Autodesk Fusion 360 part; units mm, degrees
sketch "Esquisse1" plane through (0, 0, 0) normal (0, 0, 1) x (1, 0, 0)
  line L0 (-30, 40) -> (30, 40)
  line L1 (30, 40) -> (30, -40)
  line L2 (30, -40) -> (-30, -40)
  line L3 (-30, -40) -> (-30, 40)
  line L4 (-30, 40) -> (30, -40) construction
  line L5 (30, 40) -> (-30, -40) construction
  dimension "d1" = 60
  dimension "d2" = 80
extrude "Extrusion1" add sketch "Esquisse1" along normal blind 5
sketch "Esquisse2" plane through (0, 0, 5) normal (0, 0, 1) x (-1, 0, 0)
  line L0 (30, 40) -> (-30, 40)
  line L1 (-30, 40) -> (-30, -40)
  line L2 (-30, -40) -> (30, -40)
  line L3 (30, -40) -> (30, 40)
  line L4 (4.5, -29.5) -> (-4.5, -29.5)
  line L5 (-4.5, -29.5) -> (-4.5, 29.5)
  line L6 (-4.5, 29.5) -> (4.5, 29.5)
  line L7 (4.5, 29.5) -> (4.5, -29.5)
  line L8 (4.5, -29.5) -> (-4.5, 29.5) construction
  line L9 (-4.5, -29.5) -> (4.5, 29.5) construction
  dimension "d5" = 59
  dimension "d6" = 9
extrude "Extrusion2" add sketch "Esquisse2" along normal blind 17 contours L4 L5 L6 L7
sketch "Esquisse3" plane through (0, 0, 22) normal (0, 0, 1) x (-1, 0, 0)
  line L0 (4.5, 29.5) -> (-4.5, 29.5)
  line L1 (-4.5, 29.5) -> (-4.5, -29.5)
  line L2 (-4.5, -29.5) -> (4.5, -29.5)
  line L3 (4.5, -29.5) -> (4.5, 29.5)
  line L4 (9.5, -29.5) -> (-9.5, -29.5)
  line L5 (-9.5, -29.5) -> (-9.5, 29.5)
  line L6 (-9.5, 29.5) -> (9.5, 29.5)
  line L7 (9.5, 29.5) -> (9.5, -29.5)
  line L8 (9.5, -29.5) -> (-9.5, 29.5) construction
  line L9 (-9.5, -29.5) -> (9.5, 29.5) construction
  dimension "d9" = 59
  dimension "d10" = 19
extrude "Extrusion3" add sketch "Esquisse3" along normal blind 3
sketch "Esquisse4" plane through (0, 0, 25) normal (0, 0, 1) x (-1, 0, 0)
  line L0 (9.5, 29.5) -> (-9.5, 29.5)
  line L1 (-9.5, 29.5) -> (-9.5, -29.5)
  line L2 (-9.5, -29.5) -> (9.5, -29.5)
  line L3 (9.5, -29.5) -> (9.5, 29.5)
  line L4 (-9.5, 29.5) -> (9.5, 29.5)
  line L5 (9.5, 29.5) -> (9.5, 19.5)
  line L6 (9.5, 19.5) -> (-9.5, 19.5)
  line L7 (-9.5, 19.5) -> (-9.5, 29.5)
  dimension "d13" = 10
extrude "Extrusion4" add sketch "Esquisse4" along normal blind 10 from surface at -7.5 contours L0 L1 L3 L4 L5 L6 L7
chamfer "Chanfrein5" distance 4 angle 45 1 edges at (4.5, 0, 5)
chamfer "Chanfrein6" distance 4 angle 45 1 edges at (-4.5, 0, 5)
sketch "Esquisse10" plane through (0, -29.5, 0) normal (0, -1, 0) x (1, 0, 0)
  line L0 (9.5, 17.5) -> (9.5, 27.5)
  line L1 (-9.5, 27.5) -> (-9.5, 17.5)
  line L2 (-4.5, 17.5) -> (-4.5, 9)
  line L3 (-4.5, 9) -> (-8.5, 5)
  line L4 (-8.5, 5) -> (8.5, 5)
  line L5 (8.5, 5) -> (4.5, 9)
  line L6 (4.5, 9) -> (4.5, 17.5)
  line L7 (0, 25) -> (0, 23)
  line L8 (0, 23) -> (-3.25, 23)
  line L9 (-3.25, 23) -> (3.25, 23)
  line L10 (3.25, 23) -> (3.25, 14.5)
  line L11 (3.25, 14.5) -> (-3.25, 14.5)
  line L12 (-3.25, 14.5) -> (-3.25, 23)
  line L13 (-3.25, 23) -> (3.25, 23)
  line L14 (3.25, 23) -> (3.25, 19.5)
  line L15 (3.25, 19.5) -> (-3.25, 19.5)
  line L16 (-3.25, 19.5) -> (-3.25, 23)
  line L17 (4.5, 17.5) -> (9.5, 17.5)
  line L18 (9.5, 27.5) -> (-9.5, 27.5)
  line L19 (-9.5, 27.5) -> (9.5, 27.5)
  line L20 (-9.5, 17.5) -> (-4.5, 17.5)
  point P0 (0, 25)
  point P1 (0, 23)
  dimension "d33" = 6.5
  dimension "d34" = 3.5
  dimension "d35" = 8.5
  dimension "d46" = 4.5
extrude "Extrusion9" add sketch "Esquisse10" along normal blind 6 contours L8 L9 L10 L12 L13 L14 L15 L16
extrude "Extrusion10" add sketch "Esquisse10" along normal blind 4 from surface at 5 contours L8 L9 L10 L12 L13 L14 L15 L16 | L10 L11 L12 L15
extrude "Extrusion11" add 2 faces at (7.8333, 13.1667, 22) (-7.8333, 13.1667, 22) along direction (0, 0, -1) blind 4
sketch "Esquisse11" plane through (0, 0, 5) normal (0, 0, 1) x (-1, 0, 0)
  line L0 (8.5, -29.5) -> (-8.5, -29.5)
  line L1 (-8.5, -29.5) -> (-8.5, 29.5)
  line L2 (-8.5, 29.5) -> (8.5, 29.5)
  line L3 (8.5, 29.5) -> (8.5, -29.5)
  line L4 (30, 40) -> (-30, 40)
  line L5 (-30, 40) -> (-30, -40)
  line L6 (-30, -40) -> (30, -40)
  line L7 (30, -40) -> (30, 40)
  circle A0 centre (19, -19) radius 1.55
  circle A1 centre (19, 18) radius 1.55
  circle A2 centre (-19, -19) radius 1.55
  circle A3 centre (-19, 18) radius 1.55
  dimension "d47" = 3.1
  dimension "d48" = 3.1
  dimension "d49" = 3.1
  dimension "d50" = 3.1
  dimension "d51" = 37
  dimension "d52" = 37
  dimension "d53" = 11
  dimension "d54" = 11
  dimension "d55" = 11
  dimension "d56" = 11
  dimension "d57" = 22
  dimension "d58" = 22
extrude "Extrusion12" cut sketch "Esquisse11" against normal blind 10 contours A0 | A1 | A2 | A3
chamfer "Chanfrein7" distance 1.5 angle 45 4 edges at (-17.5549, 18.4395, 5) (-17.5549, -18.5605, 5) (20.4451, 18.4395, 5) (20.4451, -18.5605, 5)
Verification items for the finished model (mm, model axes). A direction names the side the tool comes from. Round coordinates to 2 decimals unless told otherwise and drop trailing zeros. Loops run counter-clockwise (first coordinate to the right, second up) from the corner with the lowest first, then second, coordinate; pieces in that order, holes last. Notation, with made-up numbers: (58, 35.5) - (75, 35.5) arc R21 cw to (75, 47.5) - close; hole circle Ø10 at (44.25, 77). An arc over 180 degrees is marked (long way). Use a Markdown table: item, result. Add a question column.
1. Section check A-A, the plane x = 6.5. Record the boundary of the cut face in (y, z).
2. Thickness scan on probe 1 along X at (y, z) = (19, 1); probe 2 along Y at (x, z) = (-19, 1.35); probe 3 along Y at (x, z) = (0, 5.5). Record the ranges inside material, lowest first. Write a range as [from, to].
3. Release check for a two-part mould opening along X. For faces 1 (the face through (-19.83, 17.69, 1.77)), 2 (the face through (0, -32, 19.5)), 3 (the face through (6.5, 0.4, 7)), 4 (the face through (-30, -1, 2)) record: released by +X, released by -X, zero draft, split by the parting line, or undercut.
4. Section check B-B, the plane z = 15.5. Record the boundary of the cut face in (x, y), plus the area to 3 significant figures.
5. Section check D-D, the plane x = 19. Record the boundary of the cut face in (y, z), plus the area to 4 significant figures.
6. Section check C-C, the plane y = -18. Record the boundary of the cut face in (x, z).
7. Gauge pin test, flat ends, axial feed: pin 1 (18 mm diameter, centred on x = -4, y = 11, fed in from +Z); pin 2 (3.5 mm diameter, centred on x = -19, y = 19, fed in from +Z); pin 3 (5 mm diameter, centred on y = 22, z = 13, fed in from +X); pin 4 (8 mm diameter, centred on x = -1, y = 13, fed in from -Z). Record the tip position at first contact, or that the pin passes through.
8. Access from +Z, -Z, +X, -X, +Y, -Y to the whole of each face (thin tool, end or side, straight path). Record for faces 5 (the face through (0, -36, 14.5)), 6 (the face through (-7, -25, 17.5)), 7 (the face through (0, 29.5, 15)).
Checks:
| question | item | result |
|---|---|---|
| 1 | outline | (-40, 0) - (40, 0) - (40, 5) - (29.5, 5) - (29.5, 7) - (-29.5, 7) - (-29.5, 5) - (-40, 5) - close; (-29.5, 17.5) - (-19.5, 17.5) - (-19.5, 18) - (29.5, 18) - (29.5, 25) - (-19.5, 25) - (-19.5, 27.5) - (-29.5, 27.5) - close |
| 2 | probe 1 | x = [-30, -20.55], [-17.45, 17.45], [20.55, 30] |
| 2 | probe 2 | y = [-40, -19.55], [-16.45, 17.45], [20.55, 40] |
| 2 | probe 3 | y = [-29.5, 29.5] |
| 3 | face 1 | undercut |
| 3 | face 2 | zero draft |
| 3 | face 3 | released by +X |
| 3 | face 4 | released by -X |
| 4 | outline | (-4.5, -29.5) - (4.5, -29.5) - (4.5, 29.5) - (-4.5, 29.5) - close; (-3.25, -38.5) - (3.25, -38.5) - (3.25, -34.5) - (-3.25, -34.5) - close |
| 4 | area | 557 mm^2 |
| 5 | outline | (-40, 0) - (-19.55, 0) - (-19.55, 3.5) - (-21.05, 5) - (-40, 5) - close; (-16.45, 0) - (17.45, 0) - (17.45, 3.5) - (15.95, 5) - (-14.95, 5) - (-16.45, 3.5) - close; (20.55, 0) - (40, 0) - (40, 5) - (22.05, 5) - (20.55, 3.5) - close |
| 5 | area | 364.5 mm^2 |
| 6 | outline | (-30, 0) - (-20.55, 0) - (-20.55, 3.5) - (-22.05, 5) - (-30, 5) - close; (-17.45, 0) - (17.45, 0) - (17.45, 3.5) - (15.95, 5) - (8.5, 5) - (4.5, 9) - (4.5, 18) - (9.5, 18) - (9.5, 25) - (-9.5, 25) - (-9.5, 18) - (-4.5, 18) - (-4.5, 9) - (-8.5, 5) - (-15.95, 5) - (-17.45, 3.5) - close; (20.55, 0) - (30, 0) - (30, 5) - (22.05, 5) - (20.55, 3.5) - close |
| 7 | pin 1 | stops at z = 25 |
| 7 | pin 2 | stops at z = 3.7 |
| 7 | pin 3 | stops at x = 4.5 |
| 7 | pin 4 | stops at z = 0 |
| 8 | face 5 | +X, -X, -Y |
| 8 | face 6 | -X, +Y, -Y |
| 8 | face 7 | +Z, +X, -X, +Y |
